Could you check a few things on this model? Use its own coordinates, in mm. A direction names the side the tool comes from. Round coordinates to 2 decimals unless told otherwise and drop trailing zeros. Loops run counter-clockwise (first coordinate to the right, second up) from the corner with the lowest first, then second, coordinate; pieces in that order, holes last. Notation, with made-up numbers: (16.5, 43.5) -> (48.5, 43.5) arc R20 cw to (48.5, 75.5) -> close; hole circle Ø10 at (70.5, 12). An arc over 180 degrees is marked (long way). One line per item, written item: value.
from build123d import *

# Parameters (mm, degrees)
SKETCH1_R           = 25
SKETCH1_R_2         = 15
SKETCH1_R_3         = 7.5
BOSS_EXTRUDE1_DEPTH = 10
SKETCH1_3_R         = 25
SKETCH1_3_R_2       = 15
SKETCH1_3_R_3       = 7.5
BOSS_EXTRUDE2_DEPTH = 20
CUT_EXTRUDE1_DEPTH  = 20


with BuildPart() as part:
    # Sketch1 → Boss-Extrude1 (new body)
    # profile 1 of 3: a face of its own
    with BuildSketch(Plane(origin=(0, 0, 0), x_dir=(1, 0, 0), z_dir=(0, 1, 0))):
        Circle(SKETCH1_R)
        with Locations(Location((0, 0, 0), (0, 0, 270))):
            Circle(SKETCH1_R_2, mode=Mode.SUBTRACT)
    # profile 2 of 3: a face of its own
    with BuildSketch(Plane(origin=(0, 0, 0), x_dir=(1, 0, 0), z_dir=(0, 1, 0))):
        with Locations((80, 0)):
            Circle(SKETCH1_R_2)
        with Locations(Location((80, 0, 0), (0, 0, 270))):
            Circle(SKETCH1_R_3, mode=Mode.SUBTRACT)
    # profile 3 of 3: a face of its own
    with BuildSketch(Plane(origin=(0, 0, 0), x_dir=(1, 0, 0), z_dir=(0, 1, 0))):
        with BuildLine():
            Line((81.875, 14.882351125), (3.125, 24.803918541))
            ThreePointArc((3.125, 24.803918541), (18.75, 16.535945694), (25, 0))
            ThreePointArc((25, 0), (18.75, -16.535945694), (3.125, -24.803918541))
            Line((3.125, -24.803918541), (81.875, -14.882351125))
            ThreePointArc((81.875, -14.882351125), (65, 0), (81.875, 14.882351125))
        make_face()
    extrude(amount=BOSS_EXTRUDE1_DEPTH)

    # Sketch1_3 → Boss-Extrude2 (add)
    # profile 1 of 2: a face of its own
    with BuildSketch(Plane(origin=(0, 0, 0), x_dir=(1, 0, 0), z_dir=(0, 1, 0))):
        with Locations(Location((0, 0, 0), (0, 0, 82.819244219))):
            Circle(SKETCH1_3_R)
        with Locations(Location((0, 0, 0), (0, 0, 270))):
            Circle(SKETCH1_3_R_2, mode=Mode.SUBTRACT)
    # profile 2 of 2: a face of its own
    with BuildSketch(Plane(origin=(0, 0, 0), x_dir=(1, 0, 0), z_dir=(0, 1, 0))):
        with Locations(Location((80, 0, 0), (0, 0, 82.819244219))):
            Circle(SKETCH1_3_R_2)
        with Locations(Location((80, 0, 0), (0, 0, 270))):
            Circle(SKETCH1_3_R_3, mode=Mode.SUBTRACT)
    extrude(amount=BOSS_EXTRUDE2_DEPTH)

    # Sketch2 → Cut-Extrude1 (cut)
    with BuildSketch(Plane(origin=(0, 10, 0), x_dir=(1, 0, 0), z_dir=(0, 1, 0))):
        with BuildLine():
            Line((36.494317712, -12.536537589), (54.252640976, -10.299199158))
            ThreePointArc((54.252640976, -10.299199158), (57.044014201, -8.603645506), (57.641138609, -5.392709644))
            ThreePointArc((57.641138609, -5.392709644), (57, 0), (57.641138609, 5.392709644))
            ThreePointArc((57.641138609, 5.392709644), (57.044014201, 8.603645506), (54.252640976, 10.299199158))
            Line((54.252640976, 10.299199158), (36.494317712, 12.536537589))
            ThreePointArc((36.494317712, 12.536537589), (33.016873839, 11.239020501), (32.103040122, 7.641650015))
            ThreePointArc((32.103040122, 7.641650015), (33, 0), (32.103040122, -7.641650015))
            ThreePointArc((32.103040122, -7.641650015), (33.016873839, -11.239020501), (36.494317712, -12.536537589))
        make_face()
    extrude(amount=-CUT_EXTRUDE1_DEPTH, mode=Mode.SUBTRACT)


solid = part.part
(1) For faces 4 (the face through (-25, 12, 0)), 5 (the face through (45.5, 5.1, -11.4)), 6 (the face through (21, 0, 0)), which set-ups out of +Z, -Z, +X, -X, +Y, -Y let a thin tool reach every point of the face, with its end or its side?
Recorded:
face 4: +Y
face 5: +Y, -Y
face 6: +Z, -Z, +X, -X, -Y
(2) I'm going to push flat-ended pins straight in: pin 1 Ø4 at (x, z) = (72, 18.5) entering from +Y; pin 2 Ø2 at (x, z) = (45, -13.5) entering from +Y; pin 3 Ø6 at (y, z) = (14, -13) entering from +X; pin 4 Ø10 at (x, y) = (27, 14) entering from -Z. Where does each tip first touch, or does it pass through?
Recorded:
pin 1: through
pin 2: y = 10
pin 3: x = 91.18
pin 4: z = -22.17
(3) If we section it at C-C, the plane z = 0: Please give me the cut outline in (x, y), then the cut area to 3 significant figures.
Recorded:
outline: (-25, 0) -> (-15, 0) -> (-15, 20) -> (-25, 20) -> close; (15, 0) -> (33, 0) -> (33, 10) -> (25, 10) -> (25, 20) -> (15, 20) -> close; (57, 0) -> (72.5, 0) -> (72.5, 20) -> (65, 20) -> (65, 10) -> (57, 10) -> close; (87.5, 0) -> (95, 0) -> (95, 20) -> (87.5, 20) -> close
area: 860 mm²
(4) Thinking about a two-plate mould opening in Z: for faces 1 (the face through (41.949, 4.93, 19.913)), 2 (the face through (31, 10, -2)), 3 (the face through (0.66, 9.86, -14.985)), which applies, released by +Z, released by -Z, zero draft, split by the parting line, or undercut?
Recorded:
face 1: released by +Z
face 2: zero draft
face 3: undercut
(5) If we section it at D-D, the plane y = 6.75: Please give me the cut outline in (x, z) (3 decimals).
Recorded:
outline: (3.125, -24.804) -> (81.875, -14.882) arc R15 ccw to (81.875, 14.882) -> (3.125, 24.804) arc R25 ccw (long way) to start; hole circle Ø30 at (0, 0); hole (32.103, -7.642) arc R4 ccw to (36.494, -12.537) -> (54.253, -10.299) arc R4 ccw to (57.641, -5.393) arc R23 cw to (57.641, 5.393) arc R4 ccw to (54.253, 10.299) -> (36.494, 12.537) arc R4 ccw to (32.103, 7.642) arc R33 cw to start; hole circle Ø15 at (80, 0)
(6) If we section it at B-B, the plane y = 13.25: Please give me the cut outline in (x, z) (3 decimals), then the cut area to 3 significant figures.
Recorded:
outline: circle Ø50 at (0, 0); circle Ø30 at (80, 0); hole circle Ø30 at (0, 0); hole circle Ø15 at (80, 0)
area: 1,790 mm²
(7) If we section it at A-A, the plane x = 0: Please give me the cut outline in (y, z).
Recorded:
outline: (0, -25) -> (20, -25) -> (20, -15) -> (0, -15) -> close; (0, 15) -> (20, 15) -> (20, 25) -> (0, 25) -> close
(8) If I drill on L1, parallel to X at y = 10.5, z = 0; L2, parallel to X at y = 8.5, z = 2; L3, parallel to Z at x = 37.5, y = 5.25, over which ranges is the centre line in solid material (lowest first)?
Recorded:
L1: -25 to -15, 15 to 25, 65 to 72.5, 87.5 to 95
L2: -24.92 to -14.87, 14.87 to 32.94, 57.09 to 72.77, 87.23 to 94.87
L3: -20.47 to -12.41, 12.41 to 20.47
